Geometry: see drawing. Coordinates: mm, zero at the bounding-box minimum. A direction names the side the tool comes from. Round coordinates to 2 decimals unless told otherwise and drop trailing zeros. Loops run counter-clockwise (first coordinate to the right, second up) from the corner with the lowest first, then second, coordinate; pieces in that order, holes last. Notation, with made-up numbers: (-39.5, -30) -> (-9.5, -30) arc R29 ccw to (-9.5, 9) -> close; hole circle Ø5 at (74.5, -0.5). An arc over 180 degrees is marked (long way). Write item = value, one per line.
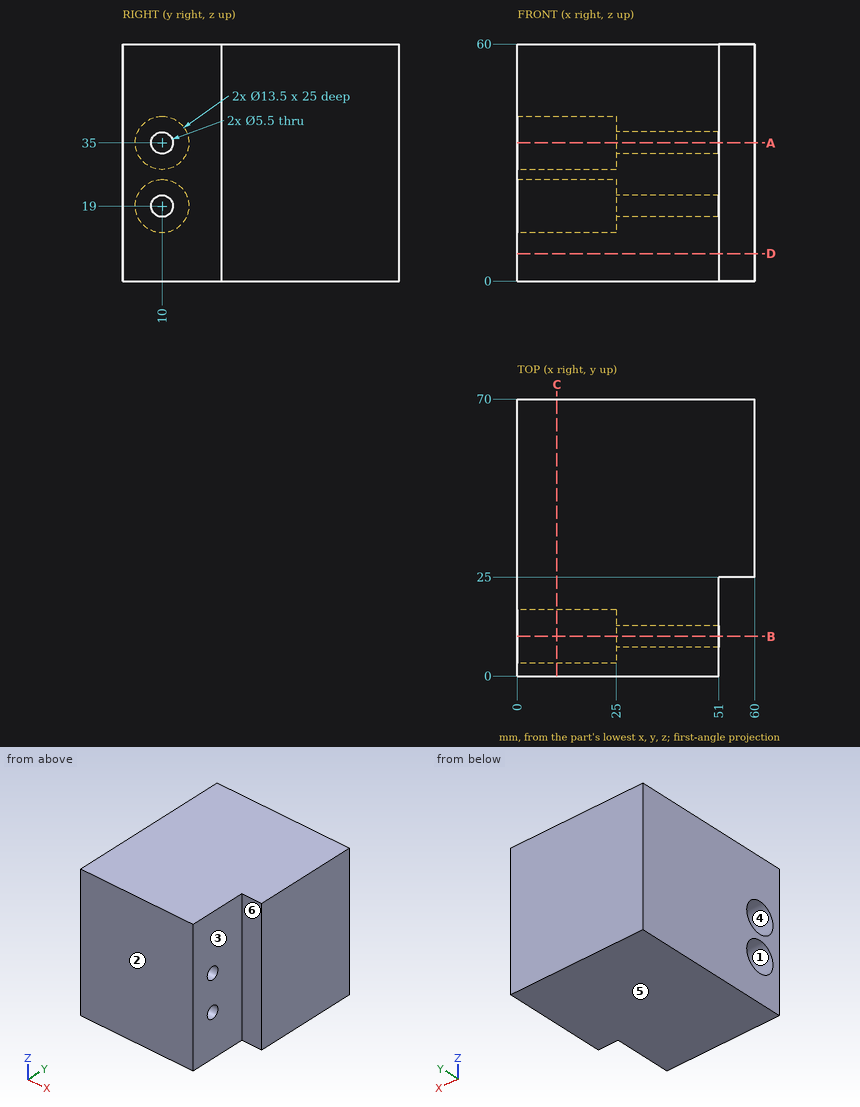
1. Contact query for flat-ended pins moving along their axis: pin 1 Ø17.5 at (y, z) = (10, 35) entering from +X; pin 2 Ø4.5 at (x, z) = (54.5, 21) entering from -Y. Output: stop coordinate, or through.
Evaluation:
pin_1 = 51
pin_2 = 25
2. Section query B-B (y = 10). Return the cut outline in (x, z), then the cut area to 3 significant figures.
Evaluation:
outline = (0, 0) -> (51, 0) -> (51, 16.25) -> (25, 16.25) -> (25, 12.25) -> (0, 12.25) -> close; (0, 25.75) -> (25, 25.75) -> (25, 21.75) -> (51, 21.75) -> (51, 32.25) -> (25, 32.25) -> (25, 28.25) -> (0, 28.25) -> close; (0, 41.75) -> (25, 41.75) -> (25, 37.75) -> (51, 37.75) -> (51, 60) -> (0, 60) -> close
area = 2,100 mm²
3. Section query C-C (x = 10). Return the cut outline in (y, z), then the cut area to 3 significant figures.
Evaluation:
outline = (0, 0) -> (70, 0) -> (70, 60) -> (0, 60) -> close; hole circle Ø13.5 at (10, 19); hole circle Ø13.5 at (10, 35)
area = 3,910 mm²
4. Set-up query: the marked faces 1, 2 and 3. Return all of +Z, -Z, +X, -X, +Y, -Y with unobstructed straight access to the full face (end or side cutting, diameter ignored); none if empty.
Evaluation:
face_1 = -X
face_2 = +Z, -Z, +X, -X, -Y
face_3 = +Z, -Z, +X, -Y
5. Section query A-A (z = 35). Return the cut outline in (x, y).
Evaluation:
outline = (0, 0) -> (51, 0) -> (51, 7.25) -> (25, 7.25) -> (25, 3.25) -> (0, 3.25) -> close; (0, 16.75) -> (25, 16.75) -> (25, 12.75) -> (51, 12.75) -> (51, 25) -> (60, 25) -> (60, 70) -> (0, 70) -> close
6. Line query: probe 1 along Y at (x, z) = (15.75, 19); probe 2 along Y at (x, z) = (31, 35); probe 3 along X at (y, z) = (15.5, 16). Output: solid intervals per line, ascending. Write a range as from..to.
Evaluation:
probe_1 = 0..3.25, 16.75..70
probe_2 = 0..7.25, 12.75..70
probe_3 = 25..51
7. Mould query, pull axis Y, two halves, no side actions, for the marked faces 4, 5 and 6. Classes: released by +Y, released by -Y, zero draft, split by the parting line, or undercut.
Evaluation:
face_4 = undercut
face_5 = zero draft
face_6 = released by -Y
8. Section query D-D (z = 7). Return the cut outline in (x, y), then the cut area to 4 significant figures.
Evaluation:
outline = (0, 0) -> (51, 0) -> (51, 25) -> (60, 25) -> (60, 70) -> (0, 70) -> close
area = 3,975 mm²
